Can you work these out from the model? Positions are in its coordinate system, mm. A direction names the side the tool comes from. Give positions to 0.01 mm unless a question says otherwise; leave off trailing zeros. Write each loop counter-clockwise with the first axis right and the second up, starting at its lowest first coordinate (ties: lowest second). Pieces come first, ordered by that corner, then holes. Notation, with made-up numbers: M 66,36 L 122,36 A22 cw 122,63 Z; hole C 70,53 d4. An arc over 180 degrees is marked long. Write each question's results on one line, items separated by ' | '.
from build123d import *

# Parameters (mm, degrees)
BOX_W          = 5
BOX_H          = 20
BOX_DEPTH      = 1
CYLINDER_R     = 2
CYLINDER_DEPTH = 20
BOX001_W       = 3
BOX001_H       = 1
BOX001_DEPTH   = 5


with BuildPart() as cube:
    # Box → Box (new body)
    with BuildSketch(Plane(origin=(3, -10, -1), x_dir=(1, 0, 0), z_dir=(0, 0, 1))):
        with Locations((2.5, 10)):
            Rectangle(BOX_W, BOX_H)
    extrude(amount=BOX_DEPTH)


with BuildPart() as fusion:
    # Cylinder → Cylinder (new body)
    with BuildSketch(Plane(origin=(0, 0, 0), x_dir=(0, 0, -1), z_dir=(1, 0, 0))):
        Circle(CYLINDER_R)
    extrude(amount=CYLINDER_DEPTH)

    # Fusion: union Cube
    add(cube.part)


with BuildPart() as aeroplane:
    # Box001 → Box001 (new body)
    with BuildSketch(Plane(origin=(0, -0.5, 0), x_dir=(1, 0, 0), z_dir=(0, 0, 1))):
        with Locations((1.5, 0.5)):
            Rectangle(BOX001_W, BOX001_H)
    extrude(amount=BOX001_DEPTH)

    # Fusion001: union Fusion
    add(fusion.part)


solid = aeroplane.part
Item 1: I want a section at D-D, the plane y = 0. Please give me the cut outline in (x, z).
Geometry says:
outline: M 0,-2 L 20,-2 L 20,2 L 3,2 L 3,5 L 0,5 Z
Item 2: I want a section at B-B, the plane y = 6.75. Please give me the cut outline in (x, z).
Geometry says:
outline: M 3,-1 L 8,-1 L 8,0 L 3,0 Z
Item 3: I want a section at A-A, the plane x = 4.75. Please give me the cut outline in (y, z).
Geometry says:
outline: M -10,-1 L -1.73,-1 A2 ccw 1.73,-1 L 10,-1 L 10,0 L 2,0 A2 ccw -2,0 L -10,0 Z
Item 4: I want a section at C-C, the plane z = 3.25. Please give me the cut outline in (x, y), and give its area (3 significant figures).
Geometry says:
outline: M 0,-0.5 L 3,-0.5 L 3,0.5 L 0,0.5 Z | area: 3.00 mm2
Item 5: For faces 1 (the face through (1, 0, 5)), 2 (the face through (1, 0.5, 3)), 3 (the face through (5, -6, -1)), 4 (the face through (5, -6, 0)), 5 (the face through (5, 6, -1)), which set-ups out of +Z, -Z, +X, -X, +Y, -Y let a thin tool reach every point of the face, with its end or its side?
Geometry says:
face 1: +Z, +X, -X, +Y, -Y | face 2: +Z, +X, -X, +Y | face 3: -Z, +X, -X, -Y | face 4: +Z, +X, -X, -Y | face 5: -Z, +X, -X, +Y
Item 6: I'm going to push flat-ended pins straight in: pin 1 (0.5 mm diameter, centred on y = -6, z = -0.5, fed in from +X); pin 2 (0.9 mm diameter, centred on x = 1.5, z = 3, fed in from -Y); pin 3 (1.5 mm diameter, centred on x = 10.5, y = 2, fed in from -Z). Where does each tip first touch, or does it pass through?
Geometry says:
pin 1: stops at x = 8 | pin 2: stops at y = -0.5 | pin 3: stops at z = -1.56
Item 7: If I drill on line 1 (Y direction, x = 5, z = 1); line 2 (Z direction, x = 6.25, y = 6.5); line 3 (Z direction, x = 4.5, y = 0), over which ranges is the centre line in solid material (lowest first)? Write a range as from..to.
Geometry says:
line 1: y = -1.73..1.73 | line 2: z = -1..0 | line 3: z = -2..2
